from build123d import *

# Parameters (mm, degrees)
SKETCH1_W             = 119.999999984
SKETCH1_H             = 25.000000005
SKETCH1_R             = 4
SKETCH1_W_2           = 34.999999984
SKETCH1_H_2           = 15.000000005
SKETCH1_W_3           = 35.000000016
BOSS_EXTRUDE1_DEPTH   = 10
FILLET1_R             = 5
M4X0_7_TAPPED_HOLE1_D = 3.3


with BuildPart() as part:
    # Sketch1 → Boss-Extrude1 (new body)
    with BuildSketch(Plane(origin=(0, 0, 0), x_dir=(1, 0, 0), z_dir=(0, 1, 0))):
        with Locations((-59.999999992, -12.500000003)):
            Rectangle(SKETCH1_W, SKETCH1_H)
        with Locations(Location((-60, -10, 0), (0, 0, 270))):
            Circle(SKETCH1_R, mode=Mode.SUBTRACT)
        with Locations((-87.499999992, -12.500000003)):
            Rectangle(SKETCH1_W_2, SKETCH1_H_2, mode=Mode.SUBTRACT)
        with Locations((-32.499999992, -12.500000003)):
            Rectangle(SKETCH1_W_3, SKETCH1_H_2, mode=Mode.SUBTRACT)
    extrude(amount=BOSS_EXTRUDE1_DEPTH)

    # Fillet1
    fillet1_edges = [part.edges().sort_by_distance(p)[0] for p in [
        (-14.999999984, 5, 20.000000005),
        (-14.999999984, 5, 5),
        (-50, 5, 5),
        (-50, 5, 20.000000005),
        (-104.999999984, 5, 5),
        (-104.999999984, 5, 20.000000005),
        (-70, 5, 20.000000005),
        (-70, 5, 5),
    ]]
    fillet(fillet1_edges, radius=FILLET1_R)

    # M4x0.7 Tapped Hole1 (through all)
    with Locations(Plane(origin=(0, 10, 0), x_dir=(1, 0, 0), z_dir=(0, 1, 0))):
        with Locations((-115, -5), (-115, -20.000000005), (-5, -5), (-5, -20.000000005)):
            Hole(M4X0_7_TAPPED_HOLE1_D / 2)


solid = part.part
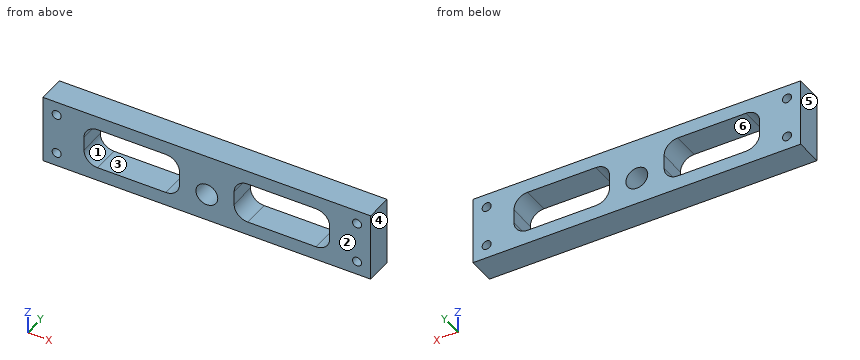
Design review of the part built by this model. Coordinates are the model's own, in mm. Face numbers are marked on the shaded views. A direction names the side the tool comes from. Give positions to 0.01 mm unless a question says otherwise; leave off trailing zeros. Write each loop counter-clockwise with the first axis right and the second up, starting at its lowest first coordinate (ties: lowest second). Pieces come first, ordered by that corner, then holes. Notation, with made-up numbers: M -39,61.25 L -5,61.25 A11 cw -5,75.25 Z; hole C -10,-20.5 d7. An arc over 180 degrees is marked long. Return JSON: item names as keys, results as strings. Group by question number.
Item 1: Take a section at A-A (x = -103). Give the boundary of the cut face in (y, z).
Item 2: Take a section at D-D (x = -60). Give the boundary of the cut face in (y, z).
Item 3: Tool access review of the marked faces 1 and 2: name each direction out of +Z, -Z, +X, -X, +Y, -Y from which nothing blocks a thin tool from reaching the whole face with its end or side.
Item 4: Clearance check with flat-ended pins moving along their axes: pin 1 Ø1.5 at (y, z) = (6.5, 12.5) entering from +X; pin 2 Ø3 at (x, z) = (-5, 5) entering from -Y. State where each tip first meets the part, or that it passes through.
Item 5: Take a section at B-B (y = 9). Give the boundary of the cut face in (x, z), plus the area to 3 significant figures.
Item 6: The part is to be moulded in two halves that separate along X. For the marked faces 3, 4, 5 and 6, say which applies: pulls with the +X half, pulls with the -X half, needs draft (parallel to the pull), parting line crosses it, or undercut.
Item 7: Wall thickness on line 1 along Z through (x, y) = (-115, 3.25); line 2 along Z through (x, y) = (-93, 7); line 3 along X through (y, z) = (5.5, 7.25): over which ranges is each line inside the solid? List them lowest first.
Item 8: Take a section at C-C (x = -5). Give the boundary of the cut face in (y, z).
Return value:
{
 "1": {"outline": "M 0,0 L 10,0 L 10,6 L 0,6 Z; M 0,19 L 10,19 L 10,25 L 0,25 Z"},
 "2": {"outline": "M 0,0 L 10,0 L 10,6 L 0,6 Z; M 0,14 L 10,14 L 10,25 L 0,25 Z"},
 "3": {"face 1": "+Y, -Y", "face 2": "+Z, -Z, +X, -X, -Y"},
 "4": {"pin 1": "stops at x = 0", "pin 2": "passes through"},
 "5": {"outline": "M -120,0 L 0,0 L 0,25 L -120,25 Z; hole C -115,5 d3.3; hole C -115,20 d3.3; hole M -105,10 A5 ccw -100,5 L -75,5 A5 ccw -70,10 L -70,15 A5 ccw -75,20 L -100,20 A5 ccw -105,15 Z; hole C -60,10 d8; hole M -50,10 A5 ccw -45,5 L -20,5 A5 ccw -15,10 L -15,15 A5 ccw -20,20 L -45,20 A5 ccw -50,15 Z; hole C -5,5 d3.3; hole C -5,20 d3.3", "area": "1,910 mm2"},
 "6": {"face 3": "undercut", "face 4": "pulls with the +X half", "face 5": "pulls with the -X half", "face 6": "undercut"},
 "7": {"line 1": "z = 0 to 3.35, 6.65 to 18.35, 21.65 to 25", "line 2": "z = 0 to 5, 20 to 25", "line 3": "x = -120 to -104.18, -70.82 to -62.9, -57.1 to -49.18, -15.82 to 0"},
 "8": {"outline": "M 0,0 L 10,0 L 10,3.35 L 0,3.35 Z; M 0,6.65 L 10,6.65 L 10,18.35 L 0,18.35 Z; M 0,21.65 L 10,21.65 L 10,25 L 0,25 Z"}
}
